Verification items for this drawing (mm, ordinates from the low corner). Coordinates: 2 decimals unless noted, no trailing zeros. Write each loop counter-clockwise with the first axis right and the second up, starting at its lowest first coordinate (ties: lowest second). Pieces come first, ordered by that corner, then holes. Notation, with made-up numbers: M 67,29 L 95,29 A22 ccw 95,52 Z; hole C -40,-18.5 d9. An arc over 180 degrees is marked long. Put each result on its own line as item: value. Start each with the question number.
1) Cross-section at D-D on x = 18. Record the cut outline in (y, z).
2) Cross-section at B-B on z = 2. Record the cut outline in (x, y), plus the area to 3 significant figures.
3) Scan lines: line 1 along Y through (x, z) = (133, 5.25); line 2 along X through (y, z) = (258, 6.25); line 3 along Y through (x, z) = (140.5, 4.75). Record each from-to range of solid material in increasing order.
4) Cross-section at A-A on y = 188. Record the cut outline in (x, z).
5) Cross-section at C-C on x = 153. Record the cut outline in (y, z), plus the area to 3 significant figures.
6) Gauge pin test, flat ends, axial feed: pin 1 (4 mm diameter, centred on x = 126, z = 3.5, fed in from -Y); pin 2 (2.5 mm diameter, centred on x = 139.5, z = 2, fed in from +Y); pin 3 (11 mm diameter, centred on x = 133, y = 188, fed in from -Z); pin 4 (4 mm diameter, centred on y = 47.5, z = 2.5, fed in from +X). Record the tip position at first contact, or that the pin passes through.
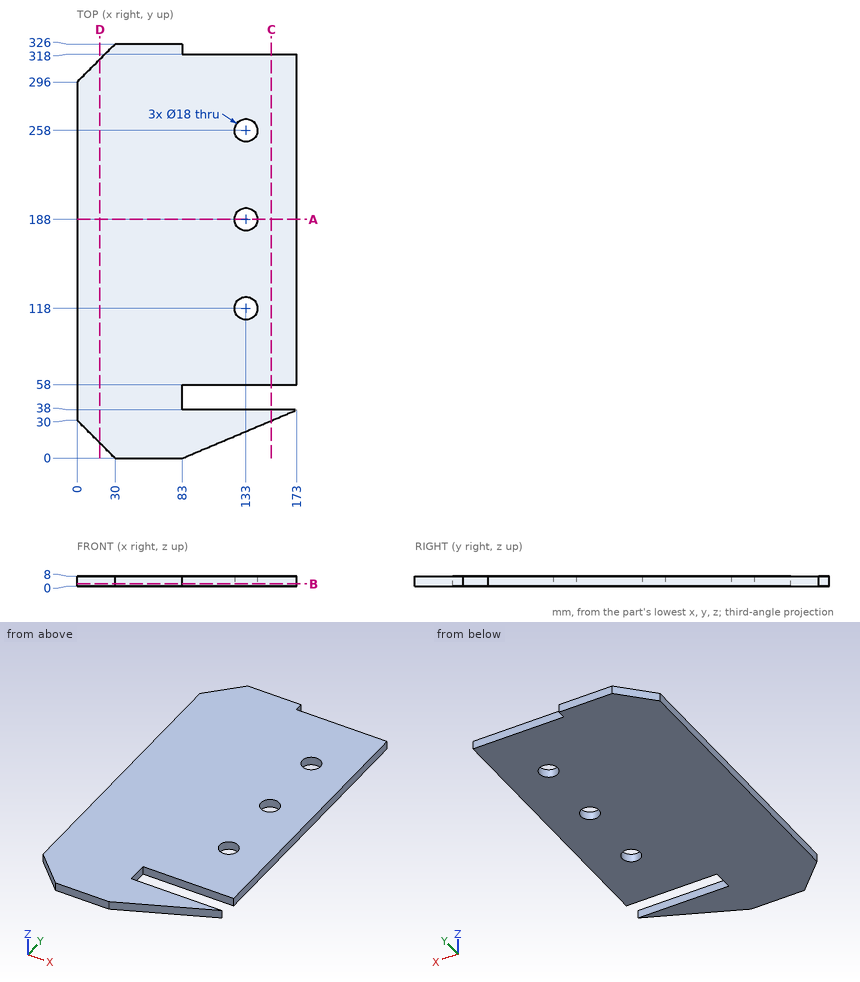
Answer key:
1. outline: M 12,0 L 314,0 L 314,8 L 12,8 Z
2. outline: M 0,30 L 30,0 L 83,0 L 173,38 L 83,38 L 83,58 L 173,58 L 173,318 L 83,318 L 83,326 L 30,326 L 0,296 Z; hole C 133,118 d18; hole C 133,188 d18; hole C 133,258 d18
2. area: 50,500 mm²
3. line 1: y = 21.11 to 38, 58 to 109, 127 to 179, 197 to 249, 267 to 318
3. line 2: x = 0 to 124, 142 to 173
3. line 3: y = 24.28 to 38, 58 to 113.03, 122.97 to 183.03, 192.97 to 253.03, 262.97 to 318
4. outline: M 0,0 L 124,0 L 124,8 L 0,8 Z; M 142,0 L 173,0 L 173,8 L 142,8 Z
5. outline: M 29.56,0 L 38,0 L 38,8 L 29.56,8 Z; M 58,0 L 318,0 L 318,8 L 58,8 Z
5. area: 2,150 mm²
6. pin 1: stops at y = 17.31
6. pin 2: stops at y = 318
6. pin 3: passes through
6. pin 4: stops at x = 83
